Input: part model. Units: mm. Frame: model coordinates. Give positions to 0.01 mm unless a question says otherwise; leave off trailing zeros. Answer as a JSON object with one key per item and string values. Group by question number.
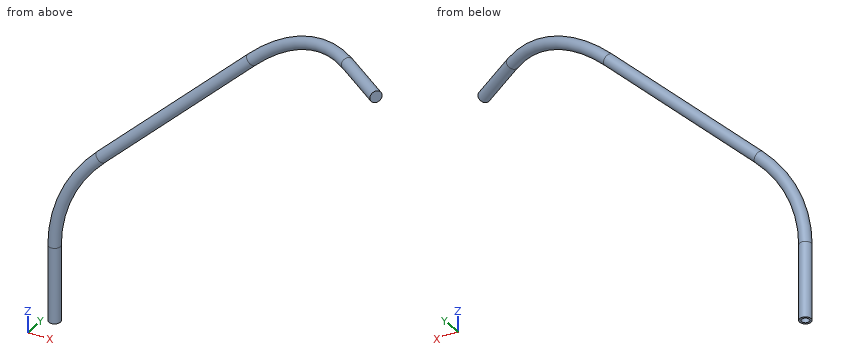
from build123d import *

# Parameters (mm, degrees)
F6_R  = 2.1844
F19_T = -0.762


with BuildPart() as f18:
    # F18: sweep along a path in F17, F15
    with BuildLine(Plane(origin=(-43.675651977, 270.5866603644, 0), x_dir=(-0.9872223923, -0.1593485118, 0), z_dir=(-0.1593485118, 0.9872223923, 0))) as f18_path:
        Line((-77.5288046302, -791.51734), (-77.5288046302, -762.7486817052))
        ThreePointArc((-77.5288046302, -762.7486817052), (-81.7230084447, -742.536315146), (-93.6130472254, -725.6615385445))
        Line((-93.6130472254, -725.6615385445), (-145.952605517, -676.668619342))
    with BuildLine(Plane(origin=(295.9948145741, 422.72440444, -384.1351665385), x_dir=(-0.8878667779, 0.3405109306, -0.3094267131), z_dir=(0.4601006245, 0.6570917897, -0.597107859))) as f18_path_2:
        ThreePointArc((220.2839333931, -303.1725531038), (196.3863531805, -293.9385533264), (171.0214128625, -297.5414541816))
        Line((171.0214128625, -297.5414541816), (150.3584973451, -306.1806072573))
    # F6 (on line) → F18 (sweep)
    with BuildSketch(Plane.XY.offset(-791.51734)):
        with Locations((32.86252, 282.94076)):
            Circle(F6_R)
    sweep(path=f18_path.line + f18_path_2.line)

    # F19
    f19_openings = [f18.faces().sort_by_distance(p)[0] for p in [
        (32.86252, 282.94076, -791.51734),
    ]]
    offset(amount=F19_T, openings=f19_openings)


solid = f18.part
1) Pin query (flat end, axial travel): P1, Ø5, axis at x = 94, y = 292, coming from the +Z side; P2, Ø2, axis at x = 118, y = 292.5, coming from the +Z side. Return the tip coordinate at first contact, or that it passes through.
2) Cut plane A-A on y = 289.5. Count the separate pieces of the cut face and the enclosed holes in it, and give its area (3 significant figures).
3) Line query: line 1 along X through (y, z) = (284, -733); line 2 along X through (y, z) = (291.5, -690); line 3 along Y through (x, z) = (101, -674). Output: solid intervals per line, ascending. Write a range as from..to.
Filled in:
{
 "1": {"P1": "stops at z = -677.61", "P2": "stops at z = -661.25"},
 "2": {"separate pieces": "2", "enclosed holes": "2", "area": "98.5 mm²"},
 "3": {"line 1": "x = 39.74..40.69, 43.98..44.96", "line 2": "x = 83.19..84.29, 88.39..89.49", "line 3": "y = 292.54..295.6"}
}
